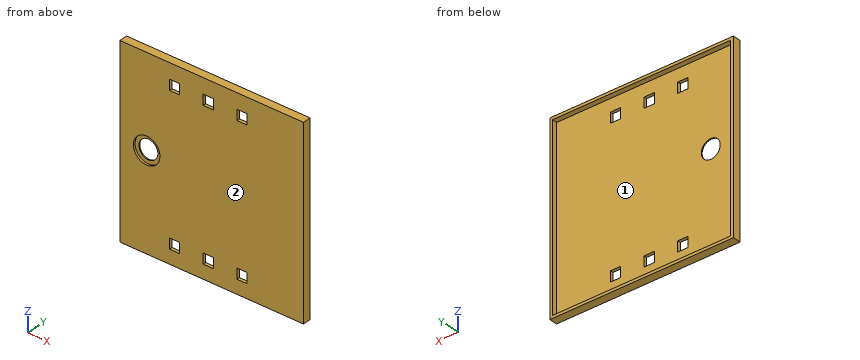
from build123d import *

# Parameters (mm, degrees)
SKETCH1_W           = 90
SKETCH1_H           = 90
BOSS_EXTRUDE1_DEPTH = 4
SKETCH2_W           = 87.35
SKETCH2_H           = 87.35
CUT_EXTRUDE2_DEPTH  = 2.5
SKETCH6_W           = 5
SKETCH6_H           = 5
CUT_EXTRUDE5_DEPTH  = 3
SKETCH7_R           = 6.5
CUT_EXTRUDE6_DEPTH  = 1
SKETCH8_R           = 4.637905468
CUT_EXTRUDE7_DEPTH  = 2.7


with BuildPart() as part:
    # Sketch1 → Boss-Extrude1 (new body)
    with BuildSketch(Plane(origin=(0, 0, 0), x_dir=(1, 0, 0), z_dir=(0, 1, 0))):
        Rectangle(SKETCH1_W, SKETCH1_H)
    extrude(amount=BOSS_EXTRUDE1_DEPTH)

    # Sketch2 → Cut-Extrude2 (cut)
    with BuildSketch(Plane(origin=(0, 4, 0), x_dir=(1, 0, 0), z_dir=(0, 1, 0))):
        Rectangle(SKETCH2_W, SKETCH2_H)
    extrude(amount=-CUT_EXTRUDE2_DEPTH, mode=Mode.SUBTRACT)

    # Sketch6 → Cut-Extrude5 (cut)
    with BuildSketch(Plane.XZ):
        with Locations((14.866822719, -35.757474477)):
            Rectangle(SKETCH6_W, SKETCH6_H)
        with Locations((-1.633815548, -35.757474477)):
            Rectangle(SKETCH6_W, SKETCH6_H)
        with Locations((-18.134453815, -35.757474477)):
            Rectangle(SKETCH6_W, SKETCH6_H)
        with Locations((14.87666148, 35.092600442)):
            Rectangle(SKETCH6_W, SKETCH6_H)
        with Locations((-1.623976787, 35.092600442)):
            Rectangle(SKETCH6_W, SKETCH6_H)
        with Locations((-18.124615054, 35.092600442)):
            Rectangle(SKETCH6_W, SKETCH6_H)
    extrude(amount=-CUT_EXTRUDE5_DEPTH, mode=Mode.SUBTRACT)

    # Sketch7 → Cut-Extrude6 (cut)
    with BuildSketch(Plane.XZ):
        with Locations((-31.818415868, 1.190037438)):
            Circle(SKETCH7_R)
    extrude(amount=-CUT_EXTRUDE6_DEPTH, mode=Mode.SUBTRACT)

    # Sketch8 → Cut-Extrude7 (cut)
    with BuildSketch(Plane.XZ.offset(-1)):
        with Locations((-31.818415868, 1.190037438)):
            Circle(SKETCH8_R)
    extrude(amount=-CUT_EXTRUDE7_DEPTH, mode=Mode.SUBTRACT)


solid = part.part
Geometry: final body of the model. Coordinates: model frame, mm. Face numbers are marked on the shaded views. Give positions to 0.01 mm unless a question says otherwise; leave off trailing zeros. Write each loop counter-clockwise with the first axis right and the second up, starting at its lowest first coordinate (ties: lowest second). Pieces come first, ordered by that corner, then holes.
(1) First-contact query: P1, Ø2, axis at x = -26, z = 29, coming from the +Y side. Flat tip, straight axial feed; report the tip coordinate or a pass-through.
(2) Cut plane B-B, the plane z = -24. Return loops of the section in (x, y) (3 decimals).
(3) Cut plane D-D, the plane z = 3. Return loops of the section in (x, y) (1 decimal), then the cut area to 3 significant figures.
(4) Cut plane C-C, the plane y = 2.9. Return loops of the section in (x, z) (3 decimals), then the cut area to 3 significant figures.
(5) Mould query, pull axis Z, two halves, no side actions, for the marked faces 1 and 2. Classes: released by +Z, released by -Z, zero draft, split by the parting line, or undercut.
(6) Ray query, line 1 (X direction, y = 0.2, z = -38); line 2 (Z direction, x = -19, y = 1.35); line 3 (Z direction, x = -23, y = 1.6) (3 decimals). Return the intervals inside material, ascending.
(7) Cut plane A-A, the plane x = -18.5. Return loops of the section in (y, z) (3 decimals).
Values follow:
1. P1: stops at y = 1.5
2. outline: (-45, 0) - (45, 0) - (45, 4) - (43.675, 4) - (43.675, 1.5) - (-43.675, 1.5) - (-43.675, 4) - (-45, 4) - close
3. outline: (-45, 0) - (-38.1, 0) - (-38.1, 1) - (-36.1, 1) - (-36.1, 1.5) - (-43.7, 1.5) - (-43.7, 4) - (-45, 4) - close; (-27.5, 1) - (-25.6, 1) - (-25.6, 0) - (45, 0) - (45, 4) - (43.7, 4) - (43.7, 1.5) - (-27.5, 1.5) - close
3. area: 125 mm2
4. outline: (-45, -45) - (45, -45) - (45, 45) - (-45, 45) - close; hole (-43.675, -43.675) - (43.675, -43.675) - (43.675, 43.675) - (-43.675, 43.675) - close
4. area: 470 mm2
5. face 1: undercut
5. face 2: zero draft
6. line 1: x = -45 to -20.63, -15.63 to -4.13, 0.87 to 12.37, 17.37 to 45
6. line 2: z = -45 to -38.26, -33.26 to 32.59, 37.59 to 45
6. line 3: z = -45 to -43.675, 43.675 to 45
7. outline: (0, -45) - (4, -45) - (4, -43.675) - (1.5, -43.675) - (1.5, -38.257) - (0, -38.257) - close; (0, -33.257) - (1.5, -33.257) - (1.5, 32.593) - (0, 32.593) - close; (0, 37.593) - (1.5, 37.593) - (1.5, 43.675) - (4, 43.675) - (4, 45) - (0, 45) - close
